Part print with two shaded views. Sizes in mm from the minimum x, y, z corner. Give positions to 0.01 mm unless a question says otherwise; leave off trailing zeros. Write each loop counter-clockwise with the first axis right and the second up, starting at its lowest first coordinate (ties: lowest second). Pieces come first, ordered by that corner, then holes.
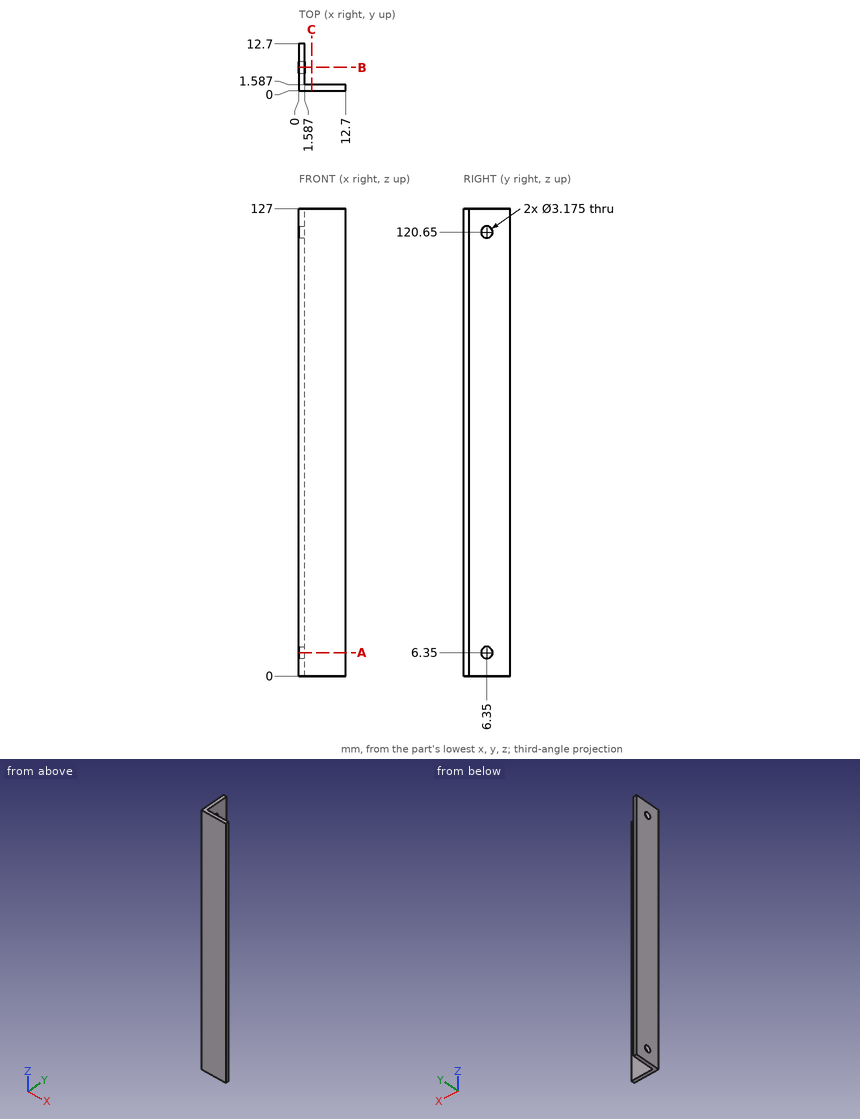
(1) Saw through at A-A, the plane z = 6.35. List the corners of the cut face in (x, y).
(2) Saw through at C-C, the plane x = 3.5. List the corners of the cut face in (y, z).
(3) Probe line 1 (Z direction, x = 0.95, y = 6.35); line 2 (Y direction, x = 0.95, z = 120.65); line 3 (Y direction, x = 2, z = 89). List the from-to ranges inside material, lowest first.
(4) Saw through at B-B, the plane y = 6.35. List the corners of the cut face in (x, z).
(5) Drop flat-ended pins along their axis: pin 1 (3 mm diameter, centred on x = 11.5, z = 74.5, fed in from +Y); pin 2 (3 mm diameter, centred on x = 2, z = 20.5, fed in from +Y). Give the stop position or say it passes through.
Computed values:
1. outline: (0, 0) - (12.7, 0) - (12.7, 1.59) - (1.59, 1.59) - (1.59, 4.76) - (0, 4.76) - close; (0, 7.94) - (1.59, 7.94) - (1.59, 12.7) - (0, 12.7) - close
2. outline: (0, 0) - (1.59, 0) - (1.59, 127) - (0, 127) - close
3. line 1: z = 0 to 4.76, 7.94 to 119.06, 122.24 to 127
3. line 2: y = 0 to 4.76, 7.94 to 12.7
3. line 3: y = 0 to 1.59
4. outline: (0, 0) - (1.59, 0) - (1.59, 4.76) - (0, 4.76) - close; (0, 7.94) - (1.59, 7.94) - (1.59, 119.06) - (0, 119.06) - close; (0, 122.24) - (1.59, 122.24) - (1.59, 127) - (0, 127) - close
5. pin 1: stops at y = 1.59
5. pin 2: stops at y = 12.7
